Source: CAD feature listing. Evaluate the final solid. Frame: model axes, mm. Coordinates: 2 decimals unless noted, no trailing zeros. Put each result on its own line as item: value.
from build123d import *

# Parameters (mm, degrees)
SKETCH_1_W        = 340
SKETCH_1_H        = 250
SKETCH_1_R        = 13
EXTRUDE_406_DEPTH = 14
CHAMFER_1_SIZE    = 2


with BuildPart() as part:
    # 草图1 → Extrude 406 (new body)
    with BuildSketch(Plane.XY):
        Rectangle(SKETCH_1_W, SKETCH_1_H)
        with Locations((-120, 80)):
            Circle(SKETCH_1_R, mode=Mode.SUBTRACT)
        with Locations((-40, 80)):
            Circle(SKETCH_1_R, mode=Mode.SUBTRACT)
        with Locations((-40, 0)):
            Circle(SKETCH_1_R, mode=Mode.SUBTRACT)
        with Locations((-120, 0)):
            Circle(SKETCH_1_R, mode=Mode.SUBTRACT)
        with Locations(Location((-40, -80, 0), (0, 0, 180))):
            Circle(SKETCH_1_R, mode=Mode.SUBTRACT)
        with Locations(Location((-120, -80, 0), (0, 0, 180))):
            Circle(SKETCH_1_R, mode=Mode.SUBTRACT)
        with Locations((120, -80)):
            Circle(SKETCH_1_R, mode=Mode.SUBTRACT)
        with Locations((40, -80)):
            Circle(SKETCH_1_R, mode=Mode.SUBTRACT)
        with Locations(Location((120, 0, 0), (0, 0, 180))):
            Circle(SKETCH_1_R, mode=Mode.SUBTRACT)
        with Locations(Location((40, 0, 0), (0, 0, 180))):
            Circle(SKETCH_1_R, mode=Mode.SUBTRACT)
        with Locations(Location((40, 80, 0), (0, 0, 180))):
            Circle(SKETCH_1_R, mode=Mode.SUBTRACT)
        with Locations(Location((120, 80, 0), (0, 0, 180))):
            Circle(SKETCH_1_R, mode=Mode.SUBTRACT)
    extrude(amount=EXTRUDE_406_DEPTH)

    # 倒角1
    chamfer_1_edges = [part.edges().sort_by_distance(p)[0] for p in [
        (170, 0, 14),
        (-133, 80, 0),
        (-133, 80, 14),
        (0, 125, 14),
        (-53, 80, 0),
        (-53, 80, 14),
        (-53, 0, 0),
        (-53, 0, 14),
        (-133, 0, 0),
        (-133, 0, 14),
        (-27, -80, 0),
        (-27, -80, 14),
        (-107, -80, 0),
        (-107, -80, 14),
        (107, -80, 0),
        (107, -80, 14),
        (27, -80, 0),
        (27, -80, 14),
        (-170, 0, 14),
        (133, 0, 0),
        (133, 0, 14),
        (0, 125, 0),
        (53, 0, 0),
        (53, 0, 14),
        (170, 0, 0),
        (53, 80, 0),
        (53, 80, 14),
        (0, -125, 0),
        (133, 80, 0),
        (133, 80, 14),
        (-170, 0, 0),
        (0, -125, 14),
    ]]
    chamfer(chamfer_1_edges, length=CHAMFER_1_SIZE)


solid = part.part
1. Cut plane A-A on x = -40. Count the separate pieces of the cut face and the enclosed holes in it, plus the area to 3 significant figures.
Numbers:
separate pieces: 4
enclosed holes: 0
area: 2,380 mm2
2. Ray query, line 1 along Y through (x, z) = (-40, 7.25); line 2 along X through (y, z) = (2, 4.75); line 3 along Y through (x, z) = (-31, 10.25). Return the intervals inside material, ascending.
Numbers:
line 1: y = -125 to -93, -67 to -13, 13 to 67, 93 to 125
line 2: x = -170 to -132.85, -107.15 to -52.85, -27.15 to 27.15, 52.85 to 107.15, 132.85 to 170
line 3: y = -125 to -89.38, -70.62 to -9.38, 9.38 to 70.62, 89.38 to 125
3. First-contact query: pin 1 (15.5 mm diameter, centred on x = 40, y = 0, fed in from +Z); pin 2 (1 mm diameter, centred on x = 54, y = 78, fed in from -Z). Flat tips, straight axial feed; report the tip coordinate or a pass-through.
Numbers:
pin 1: passes through
pin 2: stops at z = 0.36
4. Pull-direction query (Y, two-part tool) for faces 1 (the conical face through (42.845, 92.813, 1.875)), 2 (the flat face through (-2, 2, 14)), 3 (the flat face through (-2, -125, 7)); classes: pulls with the +Y half, pulls with the -Y half, needs draft (parallel to the pull), parting line crosses it, or undercut.
Numbers:
face 1: undercut
face 2: needs draft
face 3: pulls with the -Y half
